For this review, use the dimensioned drawing (mm, ordinates from the lowest corner) and the shaded views. Coordinates: 2 decimals unless noted, no trailing zeros. Answer as CSV lines item,"result". Start each with the question number.
Q1. For P1, Ø4.5, axis at x = 12.7, y = 28.61, coming from the +Z side, flat-tipped, find the tip position at first contact; note if it passes through.
Q2. Wall thickness on L1, parallel to Y at x = 75.5, z = 0.5; L2, parallel to Y at x = 31.75, z = 4 (1 decimal); L3, parallel to X at y = 105, z = 4.5 (1 decimal): over which ranges is each line inside the solid? List them lowest first. Write a range as [from, to].
Q3. Consider section A-A on x = 57.15. State how many separate pieces and enclosed holes the cut face has, and give its area (3 significant figures).
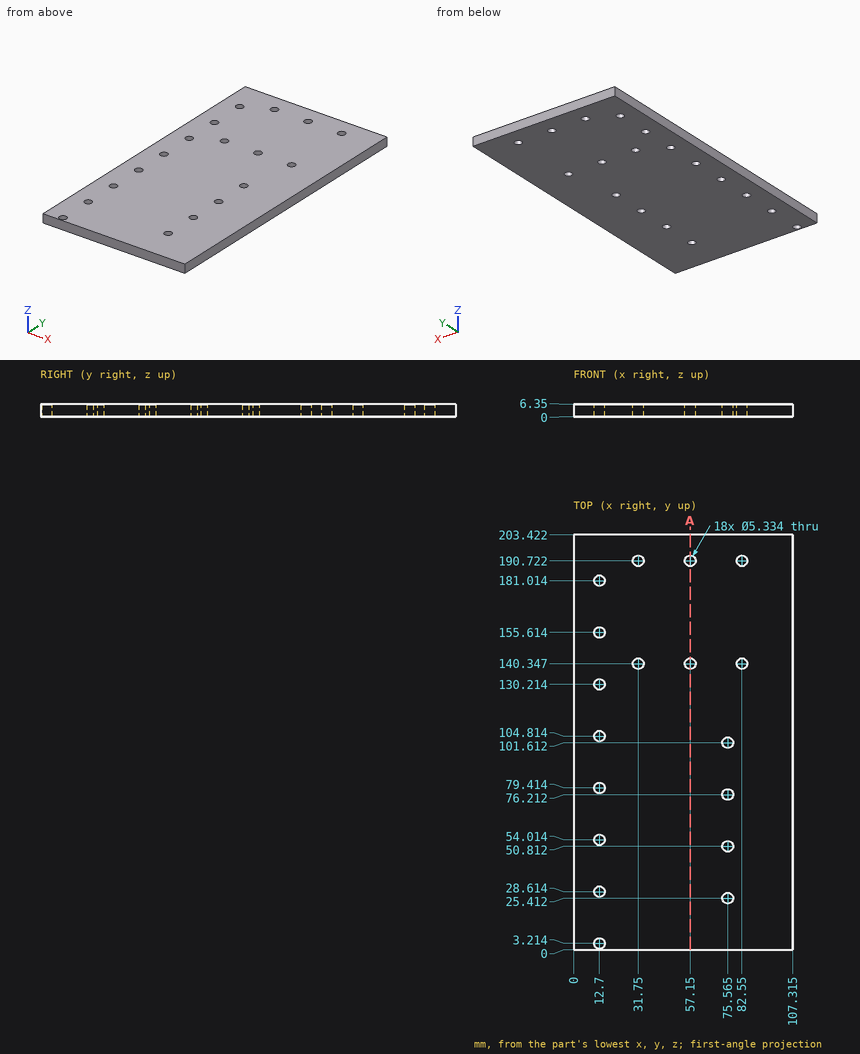
Evaluation:
1,P1,"passes through"
2,L1,"y = [0, 22.75], [28.08, 48.15], [53.48, 73.55], [78.88, 98.95], [104.28, 203.42]"
2,L2,"y = [0, 137.7], [143, 188.1], [193.4, 203.4]"
2,L3,"x = [0, 10], [15.4, 107.3]"
3,separate pieces,"3"
3,enclosed holes,"0"
3,area,"1,220 mm²"
